The model under review builds one solid part; all positions refer to its coordinate system, in mm. A direction names the side the tool comes from. Coordinates: 2 decimals unless noted, no trailing zeros. Loops run counter-clockwise (first coordinate to the right, second up) from the corner with the lowest first, then second, coordinate; pieces in that order, holes last. Notation, with made-up numbers: (13.5, -5.75) - (71.5, -5.75) arc R11 ccw to (71.5, 9.25) - close; hole circle Ø9 at (-29, 25). An arc over 180 degrees is marked (long way). One line per item, written item: value. Start each with the question number.
1. We need section A-A, the plane z = 0. Give the boundary of the cut face in (x, y), then the cut area to 4 significant figures.
2. We need section C-C, the plane z = -141. Give the boundary of the cut face in (x, y).
3. We need section B-B, the plane y = 8. Give the boundary of the cut face in (x, z).
4. We need section D-D, the plane y = 17. Give the boundary of the cut face in (x, z), then the cut area to 3 significant figures.
5. Insertion check: P1, Ø5.5, axis at x = 22.5, z = -91.5, coming from the -Y side; P2, Ø1.5, axis at x = 10, z = -44, coming from the -Y side; P3, Ø1.5, axis at x = 22.5, z = -88.5, coming from the +Y side. Each pin has a flat end and moves straight along its axis. Give the tip position at first contact, or say it passes through.
6. To check wall thickness, follow line 1 (X direction, y = -7, z = -72); line 2 (Y direction, x = -25.55, z = -180); line 3 (Y direction, x = -23, z = -26). State the ranges of each line that lie inside material, in increasing order.
7. Mouldability with a two-part tool opening along X and no side actions: class faces 1 (the face through (25.51, -0.73, 29.99)), 2 (the face through (0.35, -21.12, -88.62)), 3 (the face through (-26, 0, -59)), 4 (the face through (25, 0.4, -55.5)) as +X half, -X half, draft (parallel to the pull), parting line (faces both ways), or undercut.
8. For faces 5 (the face through (22, 0, -90)), 6 (the face through (22, -1, -93)), 7 (the face through (-25.507, -0.22, -4.995)), list the 3-axis set-ups (+Z, -Z, +X, -X, +Y, -Y) from which the entire face can be reached by the end or side of a thin tool; tool diameter is ignored.
from build123d import *

# Parameters (mm, degrees)
SKETCH1_R           = 5
SKETCH1_R_2         = 2.5
BOSS_EXTRUDE1_DEPTH = 26
CUT_EXTRUDE1_DEPTH  = 25
SKETCH5_R           = 2.67469655
SKETCH5_R_2         = 2
BOSS_EXTRUDE2_DEPTH = 1
BOSS_EXTRUDE3_START = -1
SKETCH6_R           = 2.5
SKETCH6_R_2         = 2
BOSS_EXTRUDE3_DEPTH = 1
BOSS_EXTRUDE4_START = 5
BOSS_EXTRUDE4_DEPTH = 5


with BuildPart() as part:
    # Sketch1 → Boss-Extrude1 (new, symmetric)
    with BuildSketch(Plane(origin=(0, 0, 0), x_dir=(0, 0, -1), z_dir=(1, 0, 0))):
        with BuildLine():
            Line((5.291523763, 29.529642332), (180, 14))
            ThreePointArc((180, 14), (194, 0), (180, -14))
            Line((180, -14), (5.291523763, -29.529642332))
            ThreePointArc((5.291523763, -29.529642332), (-30, 0), (5.291523763, 29.529642332))
        make_face()
        with Locations(Location((0, 0, 0), (0, 0, 180))):
            Circle(SKETCH1_R, mode=Mode.SUBTRACT)
        with Locations(Location((180, 0, 0), (0, 0, 180))):
            Circle(SKETCH1_R_2, mode=Mode.SUBTRACT)
    extrude(amount=BOSS_EXTRUDE1_DEPTH, both=True)

    # Sketch2 → Cut-Extrude1 (cut, symmetric)
    with BuildSketch(Plane(origin=(0, 0, 0), x_dir=(0, 0, -1), z_dir=(1, 0, 0))):
        with BuildLine():
            Line((5.291523763, -29.529642332), (5.114444182, -28.541439895))
            Line((5.114444182, -28.541439895), (174.506520913, -13.484366408))
            Line((174.506520913, -13.484366408), (174.595060704, -14.480439049))
            Line((174.595060704, -14.480439049), (180, -14))
            ThreePointArc((180, -14), (194, 0), (180, 14))
            Line((180, 14), (5.291523763, 29.529642332))
            ThreePointArc((5.291523763, 29.529642332), (-30, 0), (5.291523763, -29.529642332))
        make_face()
    extrude(amount=CUT_EXTRUDE1_DEPTH, both=True, mode=Mode.SUBTRACT)

    # Sketch5 → Boss-Extrude2 (add)
    with BuildSketch(Plane.ZY.offset(26)):
        with Locations((-180, 0)):
            Circle(SKETCH5_R)
        with Locations((-180, 0)):
            Circle(SKETCH5_R_2, mode=Mode.SUBTRACT)
    extrude(amount=-BOSS_EXTRUDE2_DEPTH)

    # Sketch6 → Boss-Extrude3 (add)
    with BuildSketch(Plane(origin=(26, 0, 0), x_dir=(0, 0, -1), z_dir=(1, 0, 0)).offset(BOSS_EXTRUDE3_START)):
        with Locations((180, 0)):
            Circle(SKETCH6_R)
        with Locations(Location((180, 0, 0), (0, 0, 180))):
            Circle(SKETCH6_R_2, mode=Mode.SUBTRACT)
    extrude(amount=BOSS_EXTRUDE3_DEPTH)

    # Sketch7 → Boss-Extrude4 (add)
    with BuildSketch(Plane.ZY.offset(-25).offset(BOSS_EXTRUDE4_START)):
        with BuildLine():
            Line((-5, 0), (-178, 0))
            ThreePointArc((-178, 0), (-178.068148347, -0.51763809), (-178.267949192, -1))
            Line((-178.267949192, -1), (-4.898979486, -1))
            ThreePointArc((-4.898979486, -1), (-4.974680765, -0.50254481), (-5, 0))
        make_face()
    extrude(amount=-BOSS_EXTRUDE4_DEPTH)


solid = part.part
Findings below:
1. outline: (-26, -30) - (-25, -30) - (-25, -5) - (-26, -5) - close; (-26, 5) - (-25, 5) - (-25, 30) - (-26, 30) - close; (25, -30) - (26, -30) - (26, -5) - (25, -5) - close; (25, 5) - (26, 5) - (26, 30) - (25, 30) - close
1. area: 100.0 mm2
2. outline: (-26, -17.47) - (26, -17.47) - (26, 17.47) - (25, 17.47) - (25, 0) - (20, 0) - (20, -1) - (25, -1) - (25, -16.46) - (-25, -16.46) - (-25, 17.47) - (-26, 17.47) - close
3. outline: (-26, -191.49) - (-25, -191.49) - (-25, 28.91) - (-26, 28.91) - close; (25, -191.49) - (26, -191.49) - (26, 28.91) - (25, 28.91) - close
4. outline: (-26, -146.25) - (-25, -146.25) - (-25, 24.72) - (-26, 24.72) - close; (25, -146.25) - (26, -146.25) - (26, 24.72) - (25, 24.72) - close
4. area: 342 mm2
5. P1: y = -22.11
5. P2: y = -26.16
5. P3: y = 0
6. line 1: -26 to -25, 25 to 26
6. line 2: -14 to -2, 2 to 14
6. line 3: -27.69 to -26.68
7. face 1: draft
7. face 2: undercut
7. face 3: -X half
7. face 4: undercut
8. face 5: +Z, -Z, +Y
8. face 6: +Z, -Z
8. face 7: +X, -X
